For this review, take the finished solid that the model builds, in its own axes (mm). A direction names the side the tool comes from. Give positions to 0.01 mm unless a question says otherwise; leave off trailing zeros. Write each loop counter-clockwise with the first axis right and the second up, starting at its lowest first coordinate (ties: lowest second). Pieces come first, ordered by that corner, then holes. Notation, with made-up numbers: (69.25, -24.5) -> (99.25, -24.5) arc R18 cw to (99.25, -4.5) -> close; hole circle Ø9 at (57.25, 11). An arc over 180 degrees is marked (long way). Write item = value, one per line.
```python
from build123d import *

# Parameters (mm, degrees)
SKETCH_4_W              = 17.5
SKETCH_4_H              = 11.999999999999986
SHELL_START             = 68
SHELL_1_OUTLINE_R       = 12.5
SHELL_1_DEPTH           = 17
EXTRUDE_2_REACH         = 143.612
SKETCH_7_R              = 19.99999999999999
SKETCH_8_R              = 3.500000000000001
EXTRUDE_3_DEPTH         = 8
CUT_EXTRUDE_START       = -21.159422762
CUT_EXTRUDE_1_OUTLINE_R = 15
CUT_EXTRUDE_1_DEPTH     = 21.159422762
CUT_EXTRUDE_2_REACH     = 119.224
SKETCH_9_R              = 3.0000000000000013
SKETCH_9_R_2            = 3.0000000000000018
SKETCH_9_R_3            = 2.9999999999999987
SKETCH_9_R_4            = 2.999999999999999


# Read off the part's stored shape, not the designer's step: the shell step, the extrude step
with BuildPart() as part:
    # Sketch 4 → Revolve 1 (revolve)
    with BuildSketch(Plane.XY, mode=Mode.PRIVATE) as revolve_1_sk:
        with Locations((-8.75, 79)):
            Rectangle(SKETCH_4_W, SKETCH_4_H)
        Polygon((-62.5, 8), (-62.5, 0), (-42.367966888227485, 0), (-19.99999999999999, 67.99999999999997), (0, 67.99999999999997), (0, 73.00000000000001), (-17.5, 73.00000000000001), (-23.618855180370783, 73.00000000000001), (-45, 8), align=None)
    revolve(revolve_1_sk.sketch.rotate(Axis((0, 0, 0), (0, 1, 0)), 270), axis=Axis((0, 0, 0), (0, 1, 0)))

    # Shell 1 outline → Shell 1 (cut)
    with BuildSketch(Plane(origin=(0, 0, 0), x_dir=(1, 0, 0), z_dir=(0, 1, 0)).offset(SHELL_START)):
        Circle(SHELL_1_OUTLINE_R)
    extrude(amount=SHELL_1_DEPTH, mode=Mode.SUBTRACT)

    # Sketch 7 → Extrude 2 (add, up to next)
    with BuildSketch(Plane(origin=(42.98090645471225, 14.138169005955993, 0), x_dir=(0, 0, 1), z_dir=(-0.9499276731466783, -0.31246986381111624, 0)), mode=Mode.PRIVATE) as extrude_2_sk1:
        with Locations(Location((0, 33.804881714770495, 0), (0, 0, 90))):
            Circle(SKETCH_7_R)
    extrude_2_tool1 = extrude(extrude_2_sk1.sketch, amount=EXTRUDE_2_REACH, mode=Mode.PRIVATE) - part.part


with BuildPart() as body_2:
    # Sketch 6 → Revolve 2 (revolve)
    with BuildSketch(Plane.XY):
        Polygon((32.417899669147, 46.25036163426662), (26.1685023929247, 65.24891509720017), (37.56763447068482, 68.99855346293356), (43.81703174690713, 50), align=None)
    revolve(axis=Axis((50.865675487969646, 52.31858573245586, 0), (-0.9499276731466784, -0.31246986381111624, 0)))


with BuildPart() as part_1:
    add(part.part)

    add(body_2.part)  # Extrude 2 merges body 2
    add(extrude_2_tool1.solids().sort_by_distance((32.4179, 46.250362, 0))[0])
    add(extrude_2_tool1.solids().sort_by_distance((32.4179, 46.250362, 0))[1])

    # Sketch 8 → Extrude 3 (add)
    # profile 1 of 2: a face of its own
    with BuildSketch(Plane(origin=(54.38003853247239, 17.88780737168939, 0), x_dir=(0, 0, -1), z_dir=(0.9499276731466783, 0.31246986381111624, 0))):
        with BuildLine():
            ThreePointArc((33.3333333333333, 24.37679227788569), (39.999999077050425, 33.804881714770474), (33.3333333333333, 43.23297115165526))
            Line((33.3333333333333, 43.23297115165526), (6.666667281966372, 52.66106232887043))
            ThreePointArc((6.666667281966377, 52.66106232887044), (16.329931806950803, 45.35188683213041), (19.99999999999999, 33.804881714770495))
            ThreePointArc((19.99999999999999, 33.80488171477049), (16.329931806950796, 22.257876597410572), (6.666667281966361, 14.948701100670544))
            Line((6.666667281966372, 14.948701100670537), (33.3333333333333, 24.376792277885695))
        make_face()
        with Locations(Location((30, 33.80488171477048, 0), (0, 0, 90))):
            Circle(SKETCH_8_R, mode=Mode.SUBTRACT)
    # profile 2 of 2: a face of its own
    with BuildSketch(Plane(origin=(54.38003853247239, 17.88780737168939, 0), x_dir=(0, 0, -1), z_dir=(0.9499276731466783, 0.31246986381111624, 0))):
        with BuildLine():
            ThreePointArc((-6.666667281966367, 14.948701100670544), (-19.99999999999999, 33.804881714770495), (-6.666667281966375, 52.66106232887044))
            Line((-6.666667281966372, 52.66106232887043), (-33.3333333333333, 43.23297115165526))
            ThreePointArc((-33.3333333333333, 43.23297115165526), (-39.999999077050425, 33.804881714770474), (-33.3333333333333, 24.37679227788569))
            Line((-33.3333333333333, 24.376792277885695), (-6.666667281966372, 14.948701100670537))
        make_face()
        with Locations(Location((-30, 33.80488171477048, 0), (0, 0, 90))):
            Circle(SKETCH_8_R, mode=Mode.SUBTRACT)
    extrude(amount=-EXTRUDE_3_DEPTH)

    # Cut-Extrude 1 outline → Cut-Extrude 1 (cut)
    with BuildSketch(Plane(origin=(54.38003853247239, 17.88780737168939, 0), x_dir=(0, 0, -1), z_dir=(0.9499276731466783, 0.31246986381111624, 0)).offset(CUT_EXTRUDE_START)):
        with Locations((0, 33.804881715)):
            Circle(CUT_EXTRUDE_1_OUTLINE_R)
    extrude(amount=CUT_EXTRUDE_1_DEPTH, mode=Mode.SUBTRACT)

    # Sketch 9 → Cut-Extrude 2 (cut, up to next)
    with BuildSketch(Plane(origin=(0, 8, 0), x_dir=(1, 0, 0), z_dir=(0, 1, 0)), mode=Mode.PRIVATE) as cut_extrude_2_sk1:
        with Locations(Location((-52.5, 0, 0), (0, 0, 270))):
            Circle(SKETCH_9_R)
    cut_extrude_2_tool1 = extrude(cut_extrude_2_sk1.sketch, amount=-CUT_EXTRUDE_2_REACH, mode=Mode.PRIVATE) & part_1.part
    # Sketch 9 → Cut-Extrude 2 (cut, up to next)
    with BuildSketch(Plane(origin=(0, 8, 0), x_dir=(1, 0, 0), z_dir=(0, 1, 0)), mode=Mode.PRIVATE) as cut_extrude_2_sk2:
        with Locations(Location((-26.249999999999893, 45.46633369868309, 0), (0, 0, 270))):
            Circle(SKETCH_9_R_2)
    cut_extrude_2_tool2 = extrude(cut_extrude_2_sk2.sketch, amount=-CUT_EXTRUDE_2_REACH, mode=Mode.PRIVATE) & part_1.part
    # Sketch 9 → Cut-Extrude 2 (cut, up to next)
    with BuildSketch(Plane(origin=(0, 8, 0), x_dir=(1, 0, 0), z_dir=(0, 1, 0)), mode=Mode.PRIVATE) as cut_extrude_2_sk3:
        with Locations(Location((26.25000000000021, 45.46633369868293, 0), (0, 0, 270))):
            Circle(SKETCH_9_R)
    cut_extrude_2_tool3 = extrude(cut_extrude_2_sk3.sketch, amount=-CUT_EXTRUDE_2_REACH, mode=Mode.PRIVATE) & part_1.part
    # Sketch 9 → Cut-Extrude 2 (cut, up to next)
    with BuildSketch(Plane(origin=(0, 8, 0), x_dir=(1, 0, 0), z_dir=(0, 1, 0)), mode=Mode.PRIVATE) as cut_extrude_2_sk4:
        with Locations(Location((52.5, -3.6661e-13, 0), (0, 0, 270))):
            Circle(SKETCH_9_R_2)
    cut_extrude_2_tool4 = extrude(cut_extrude_2_sk4.sketch, amount=-CUT_EXTRUDE_2_REACH, mode=Mode.PRIVATE) & part_1.part
    # Sketch 9 → Cut-Extrude 2 (cut, up to next)
    with BuildSketch(Plane(origin=(0, 8, 0), x_dir=(1, 0, 0), z_dir=(0, 1, 0)), mode=Mode.PRIVATE) as cut_extrude_2_sk5:
        with Locations(Location((26.249999999999574, -45.46633369868327, 0), (0, 0, 270))):
            Circle(SKETCH_9_R_3)
    cut_extrude_2_tool5 = extrude(cut_extrude_2_sk5.sketch, amount=-CUT_EXTRUDE_2_REACH, mode=Mode.PRIVATE) & part_1.part
    # Sketch 9 → Cut-Extrude 2 (cut, up to next)
    with BuildSketch(Plane(origin=(0, 8, 0), x_dir=(1, 0, 0), z_dir=(0, 1, 0)), mode=Mode.PRIVATE) as cut_extrude_2_sk6:
        with Locations(Location((-26.25000000000053, -45.46633369868272, 0), (0, 0, 270))):
            Circle(SKETCH_9_R_4)
    cut_extrude_2_tool6 = extrude(cut_extrude_2_sk6.sketch, amount=-CUT_EXTRUDE_2_REACH, mode=Mode.PRIVATE) & part_1.part
    add(cut_extrude_2_tool1.solids().sort_by_distance((-52.5, 8, 0))[0], mode=Mode.SUBTRACT)
    add(cut_extrude_2_tool2.solids().sort_by_distance((-26.25, 8, -45.466334))[0], mode=Mode.SUBTRACT)
    add(cut_extrude_2_tool3.solids().sort_by_distance((26.25, 8, -45.466334))[0], mode=Mode.SUBTRACT)
    add(cut_extrude_2_tool4.solids().sort_by_distance((52.5, 8, 0))[0], mode=Mode.SUBTRACT)
    add(cut_extrude_2_tool5.solids().sort_by_distance((26.25, 8, 45.466334))[0], mode=Mode.SUBTRACT)
    add(cut_extrude_2_tool6.solids().sort_by_distance((-26.25, 8, 45.466334))[0], mode=Mode.SUBTRACT)


solid = part_1.part
```
(1) The part is to be moulded in two halves that separate along Y. For faces 1 (the face through (44.47, 35.4, 20.19)), 2 (the face through (0, 73, -18)), 3 (the face through (11.923, 76.381, -3.755)), say which applies: released by +Y, released by -Y, zero draft, split by the parting line, or undercut.
Answers below:
face_1 = undercut
face_2 = released by +Y
face_3 = zero draft
(2) Take a section at D-D (y = 17.5). Write out the cut boundary in (x, z).
Answers below:
outline = circle Ø83.75 at (0, 0); hole circle Ø73.22 at (0, 0)
(3) Take a section at A-A (x = 0). Write out the cut boundary in (y, z).
Answers below:
outline = (0, -62.5) -> (8, -62.5) -> (8, -45) -> (73, -23.62) -> (73, -17.5) -> (85, -17.5) -> (85, -12.5) -> (68, -12.5) -> (68, -20) -> (0, -42.37) -> close; (0, 42.37) -> (68, 20) -> (68, 12.5) -> (85, 12.5) -> (85, 17.5) -> (73, 17.5) -> (73, 23.62) -> (8, 45) -> (8, 62.5) -> (0, 62.5) -> close
(4) To check wall thickness, follow probe 1 along Z at (x, y) = (26, 4); probe 2 along X at (y, z) = (59.5, -19); probe 3 along X at (y, z) = (76, 0). State the ranges of each line that lie inside material, in increasing order.
Answers below:
probe_1 = -56.84 to -48.46, -42.48 to -31.77, 31.77 to 42.48, 48.46 to 56.84
probe_2 = -20.65 to -12.6, 12.6 to 20.65, 32.27 to 40.69
probe_3 = -17.5 to -12.5, 12.5 to 17.5
(5) For pin 1 (20 mm diameter, centred on x = -1, z = -9.5, fed in from -Y); pin 2 (1 mm diameter, centred on x = -7.5, z = -16.5, fed in from +Y); pin 3 (1 mm diameter, centred on x = 27, y = 19.5, fed in from -Z), all flat-tipped, find the tip position at first contact; note any pin that passes through.
Answers below:
pin_1 = 68
pin_2 = 73
pin_3 = -31.62
(6) Tool access review of faces 4 (the face through (41.4, 8, 18.2)), 5 (the face through (36.19, 47.58, -25.72)), 6 (the face through (36.135, 47.751, 23.567)): name each direction out of +Z, -Z, +X, -X, +Y, -Y from which nothing blocks a thin tool from reaching the whole face with its end or side.
Answers below:
face_4 = none
face_5 = -Z
face_6 = +Z
(7) Take a section at B-B (z = 0). Count the separate pieces of the cut face and the enclosed holes in it, plus the area to 3 significant figures.
Answers below:
separate_pieces = 5
enclosed_holes = 0
area = 1,090 mm^2
